Work out the finished part from the listing and answer in its coordinate system (mm). A direction names the side the tool comes from. Round coordinates to 2 decimals unless told otherwise and drop trailing zeros. Order: outer loops, then holes, each group sorted by start corner. A loop starts at its lowest first (then second) coordinate and runs counter-clockwise, first axis right, second up. Notation, with made-up numbers: (-22.5, -11) -> (26.5, -11) arc R17 ccw to (26.5, -5) -> close; hole circle Ø10 at (-15, 62). An arc over 180 degrees is marked (long way). Use a Markdown table: item, result. Add a question column.
Item 1: Find the intervals of material crossed by L1, parallel to X at y = 33.4, z = 29; L2, parallel to Y at x = -23, z = -3; L3, parallel to Z at x = -13, y = 28, in increasing order. Write a range as [from, to].
Item 2: A cutting plane is placed at A-A, the plane y = 33.5. Determine the outline of the cut face in (x, z), plus the area to 3 significant figures.
Item 3: For a pull along Z with two mould halves and no side action, classify faces 6 (the flat face through (-21, 0, 0)), 7 (the cylindrical face through (0.438, 33.028, -24.707)), 8 (the cylindrical face through (-29.993, 2.465, 0.66)), 9 (the cylindrical face through (2, 19, 21)) as +Z half, -Z half, draft (parallel to the pull), parting line (faces both ways), or undercut.
Item 4: A cutting plane is placed at B-B, the plane x = -2. Determine the outline of the cut face in (y, z).
Item 5: A tool of negligible diameter and unlimited length cuts with its end or side. For faces 1 (the flat face through (0, 2, 26)), 2 (the cylindrical face through (-4.4, 32.97, 30.91)), 3 (the flat face through (-23, 5, -5)), 4 (the flat face through (0, 2, -27)), 5 (the cylindrical face through (-11.07, 33.03, 21.75)), from which of +Z, -Z, +X, -X, +Y, -Y can it reach the whole face along a straight path? Write none if from no direction.
Item 6: A cutting plane is placed at D-D, the plane x = -9. Determine the outline of the cut face in (y, z), plus the area to 3 significant figures.
Item 7: Flat-ended cylindrical pins translate along their axes: P1, Ø0.6, axis at y = 34, z = -28.5, coming from the +X side; P2, Ø3, axis at x = -5, z = 29, coming from the +Y side; P3, Ø6, axis at x = -26.5, y = 8.5, coming from the +Z side; P4, Ø4.5, axis at x = -18.38, z = 18.38, coming from the -Y side. Find the tip coordinate at first contact, or state that the pin passes through.
Item 8: A cutting plane is placed at C-C, the plane z = 0. Determine the outline of the cut face in (x, y).
from build123d import *

# Parameters (mm, degrees)
BOSS_EXTRUDE1_DEPTH = 38
BOSS_EXTRUDE2_DEPTH = 5
SKETCH3_R           = 2
CUT_EXTRUDE1_DEPTH  = 5
BOSS_EXTRUDE3_START = -4
BOSS_EXTRUDE3_DEPTH = 4
SKETCH5_R           = 2
CUT_EXTRUDE2_DEPTH  = 4
FILLET1_R           = 10


with BuildPart() as part:
    # Sketch1 → Boss-Extrude1 (new body)
    with BuildSketch(Plane(origin=(0, 0, 0), x_dir=(1, 0, 0), z_dir=(0, 1, 0))):
        with BuildLine():
            ThreePointArc((0, 23), (-23, 0), (0, -23))
            ThreePointArc((0, -23), (2, -21), (0, -19))
            ThreePointArc((0, -19), (-19, 0), (0, 19))
            ThreePointArc((0, 19), (2, 21), (0, 23))
        make_face()
    extrude(amount=BOSS_EXTRUDE1_DEPTH)

    # Sketch2 → Boss-Extrude2 (add)
    with BuildSketch(Plane(origin=(0, 0, 0), x_dir=(1, 0, 0), z_dir=(0, 1, 0))):
        with BuildLine():
            Line((0, 30), (0, 23))
            ThreePointArc((0, 23), (-23, 0), (0, -23))
            Line((0, -23), (0, -30))
            ThreePointArc((0, -30), (-30, 0), (0, 30))
        make_face()
    extrude(amount=BOSS_EXTRUDE2_DEPTH)

    # Sketch3 → Cut-Extrude1 (cut)
    with BuildSketch(Plane(origin=(0, 0, 0), x_dir=(-1, 0, 0), z_dir=(0, -1, 0))):
        with Locations(Location((18.384776311, -18.384776311, 0), (0, 0, 90))):
            Circle(SKETCH3_R)
    cut_extrude1 = extrude(amount=-CUT_EXTRUDE1_DEPTH, mode=Mode.SUBTRACT)

    # Mirror1: Cut-Extrude1 across plane
    add(cut_extrude1.mirror(Plane.XY), mode=Mode.SUBTRACT)

    # Sketch4 → Boss-Extrude3 (add)
    with BuildSketch(Plane(origin=(0, 35, 0), x_dir=(1, 0, 0), z_dir=(0, 1, 0)).offset(BOSS_EXTRUDE3_START)):
        with BuildLine():
            Line((0, 28.877875957), (0, 23))
            ThreePointArc((0, 23), (-5.128361746, 22.420970224), (-9.998508349, 20.713035287))
            Line((-9.998508349, 20.713035287), (-9.998508349, 29))
            ThreePointArc((-9.998508349, 29), (-4.937441773, 33.999627073), (0, 28.877875957))
        make_face()
    boss_extrude3 = extrude(amount=BOSS_EXTRUDE3_DEPTH)

    # Sketch5 → Cut-Extrude2 (cut)
    with BuildSketch(Plane.XZ.offset(-31)):
        with Locations(Location((-4.998508349, -29, 0), (0, 0, 270))):
            Circle(SKETCH5_R)
    cut_extrude2 = extrude(amount=-CUT_EXTRUDE2_DEPTH, mode=Mode.SUBTRACT)

    # Mirror2: Boss-Extrude3, Cut-Extrude2 across plane
    add(boss_extrude3.mirror(Plane.XY))
    add(cut_extrude2.mirror(Plane.XY), mode=Mode.SUBTRACT)

    # Fillet1
    fillet1_edges = [part.edges().sort_by_distance(p)[0] for p in [
        (0, 33, -23),
        (-9.998508349, 33, -20.713035287),
        (-9.998508349, 33, 20.713035287),
        (0, 33, 23),
    ]]
    fillet(fillet1_edges, radius=FILLET1_R)


solid = part.part
Reported:
| question | item | result |
|---|---|---|
| 1 | L1 | [-10, -7], [-3, 0] |
| 1 | L2 | [0, 5] |
| 1 | L3 | [-18.97, -13.86], [13.86, 18.97] |
| 2 | outline | (-13.94, -18.3) arc R10 cw to (-10, -26.25) -> (-10, -29) arc R5 ccw (long way) to (0, -28.88) -> (0, -27.63) arc R10 cw to (1.67, -22.11) arc R2 ccw to (0, -19) arc R19 cw to (0, 19) arc R2 ccw to (1.67, 22.11) arc R10 cw to (0, 27.63) -> (0, 28.88) arc R5 ccw (long way) to (-10, 29) -> (-10, 26.25) arc R10 cw to (-13.94, 18.3) arc R23 ccw to start; hole circle Ø4 at (-5, -29); hole circle Ø4 at (-5, 29) |
| 2 | area | 477 mm² |
| 3 | face 6 | draft |
| 3 | face 7 | -Z half |
| 3 | face 8 | parting line |
| 3 | face 9 | undercut |
| 4 | outline | (0, -29.93) -> (5, -29.93) -> (5, -22.91) -> (31, -22.91) -> (31, -33) -> (35, -33) -> (35, -22.91) -> (38, -22.91) -> (38, -18.89) -> (0, -18.89) -> close; (0, 18.89) -> (38, 18.89) -> (38, 22.91) -> (35, 22.91) -> (35, 33) -> (31, 33) -> (31, 22.91) -> (5, 22.91) -> (5, 29.93) -> (0, 29.93) -> close |
| 5 | face 1 | +Z, +X, -Y |
| 5 | face 2 | +Y |
| 5 | face 3 | -X |
| 5 | face 4 | -Z, +X, -Y |
| 5 | face 5 | +Z, -X, +Y |
| 6 | outline | (0, -28.62) -> (5, -28.62) -> (5, -21.17) -> (31, -21.17) -> (31, -32) -> (35, -32) -> (35, -21.17) -> (38, -21.17) -> (38, -16.73) -> (0, -16.73) -> close; (0, 16.73) -> (38, 16.73) -> (38, 21.17) -> (35, 21.17) -> (35, 32) -> (31, 32) -> (31, 21.17) -> (5, 21.17) -> (5, 28.62) -> (0, 28.62) -> close |
| 6 | area | 498 mm² |
| 7 | P1 | x = 0 |
| 7 | P2 | y = 5 |
| 7 | P3 | through |
| 7 | P4 | y = 0 |
| 8 | outline | (-30, 0) -> (-19, 0) -> (-19, 38) -> (-23, 38) -> (-23, 5) -> (-30, 5) -> close |
